Model file for the job. Use its own axes, mm. Coordinates: 2 decimals unless noted, no trailing zeros. Write each loop counter-clockwise with the first axis right and the second up, starting at its lowest first coordinate (ties: lowest second). Pieces come first, ordered by that corner, then holes. Notation, with made-up numbers: M 60,-20.5 L 72,-20.5 A24 ccw 72,9.5 Z; hole C 51,1.25 d10. An arc over 180 degrees is marked long. One line per question, with ' | ' between items. Start each with the question number.
(1) Cut at A-A (x = -267). Write the cut outline in (y, z).
(2) Flat gauge pins, fed straight in: pin 1 Ø0.8 at (x, y) = (-261.5, 1) entering from -Z; pin 2 Ø0.5 at (x, y) = (-262.5, 1) entering from +Z. Where does each tip first touch, or does it go through?
(3) Cut at C-C (z = -274). Write the cut outline in (x, y).
(4) Cut at B-B (x = -166.5). Write the cut outline in (y, z), plus the area to 3 significant figures.
(5) Wall check: probe 1 along X at (y, z) = (0.25, -95); probe 2 along Z at (x, y) = (-141.5, 0.9); probe 3 along Z at (x, y) = (-266, 0.4). Give the ranges that are in metal, low to high.
(6) Cut at D-D (y = 0.9). Count the separate pieces of the cut face and the enclosed holes in it, plus the area to 3 significant figures.
Autodesk Inventor part; units mm, degrees
ref_plane "YZ Plane" through (0, 0, 0) normal (1, 0, 0) x (0, 1, 0)
ref_plane "XZ Plane" through (0, 0, 0) normal (0, 1, 0) x (-1, 0, 0)
ref_plane "XY Plane" through (0, 0, 0) normal (0, 0, 1) x (1, 0, 0)
sketch "Sketch1" plane through (0, 0, 0) normal (0, 1, 0) x (-1, 0, 0)
  line L0 (0, 0) -> (355.6, 0)
  line L1 (355.6, 0) -> (355.6, -289.56)
  line L2 (355.6, -289.56) -> (0, -289.56)
  line L3 (0, -289.56) -> (0, 0)
  circle A0 centre (355.6, 0) radius 2.1082
  line L4 (355.6, 0) -> (361.95, 0)
  line L5 (355.6, 0) -> (355.6, 6.35)
  line L6 (355.6, 6.35) -> (361.95, 6.35)
  line L7 (0, -289.56) -> (0, -295.91)
  line L8 (0, -295.91) -> (-6.35, -295.91)
  line L9 (-6.35, -295.91) -> (361.95, -295.91)
  line L10 (361.95, -295.91) -> (361.95, 6.35)
  line L11 (361.95, 6.35) -> (-6.35, 6.35)
  line L12 (-6.35, 6.35) -> (-6.35, -295.91)
  circle A1 centre (355.6, -289.56) radius 2.1082
  circle A2 centre (0, -289.56) radius 2.1082
  circle A3 centre (0, 0) radius 2.1082
  line L13 (0, 0) -> (0, -20.32)
  line L14 (0, -20.32) -> (10.16, -20.32)
  line L15 (0, 0) -> (5.08, 0)
  line L16 (0, -289.56) -> (5.08, -289.56)
  line L17 (0, -289.56) -> (0, -269.24)
  line L18 (0, -269.24) -> (11.0826, -269.24)
  line L19 (355.6, 0) -> (355.6, -20.32)
  line L20 (355.6, -20.32) -> (345.44, -20.32)
  line L21 (355.6, 0) -> (350.52, 0)
  line L22 (355.6, -289.56) -> (350.52, -289.56)
  line L23 (355.6, -289.56) -> (355.6, -269.24)
  line L24 (355.6, -269.24) -> (345.44, -269.24)
  line L25 (345.44, -20.32) -> (10.16, -20.32)
  line L26 (355.6, -20.32) -> (355.6, -33.02)
  line L27 (355.6, -33.02) -> (0, -33.02)
  line L28 (355.6, -269.24) -> (355.6, -256.54)
  line L29 (355.6, -256.54) -> (0, -256.54)
  line L30 (345.44, -269.24) -> (11.0826, -269.24)
  line L31 (0, 0) -> (6.35, 0)
  arc A4 (6.35, 0) -> (10.16, -20.32) centre (82.4575, 3.753) ccw
  line L32 (6.35, 0) -> (-6.35, 0)
  line L33 (-6.35, 0) -> (-6.35, -289.56)
  line L34 (-6.35, -289.56) -> (6.35, -289.56)
  line L35 (6.35, -289.56) -> (6.35, 0)
  arc A5 (11.0826, -269.24) -> (6.35, -289.56) centre (82.2313, -296.5221) ccw
  line L36 (355.6, 0) -> (349.25, 0)
  line L37 (349.25, 0) -> (349.25, -289.56)
  arc A6 (349.25, -289.56) -> (345.44, -269.24) centre (298.4597, -288.566) ccw
  arc A7 (345.44, -20.32) -> (349.25, 0) centre (298.4597, -0.994) ccw
  line L38 (349.25, 0) -> (349.25, 6.35)
  line L39 (349.25, -289.56) -> (349.25, -295.91)
  line L40 (6.35, -289.56) -> (6.35, -295.91)
  line L41 (6.35, 0) -> (6.35, 6.35)
  dimension "d0" = 355.6
  dimension "d1" = 289.56
  dimension "d2" = 4.2164
  dimension "d3" = 6.35
  dimension "d4" = 6.35
  dimension "d5" = 6.35
  dimension "d6" = 6.35
  dimension "d7" = 20.32
  dimension "d8" = 10.16
  dimension "d10" = 20.32
  dimension "d12" = 20.32
  dimension "d13" = 10.16
  dimension "d16" = 5.08
  dimension "d17" = 20.32
  dimension "d18" = 10.16
  dimension "d20" = 12.7
  dimension "d21" = 12.7
  dimension "d23" = 6.35
  dimension "d24" = 76.2
  dimension "d25" = 76.2
  dimension "d26" = 6.35
  dimension "d27" = 50.8
  dimension "d28" = 50.8
extrude "Extrusion1" add sketch "Sketch1" along normal blind 1.5875 contours A3 L32 L12 L11 L41 L0 | L0 L35 L14 L3 A3 | L3 A2 L34 L12 L32 A3 | L14 L35 L27 L3 | A4 L14 L35 | L27 L35 L29 L3 | L14 L25 L20 L37 L27 L35 | L34 A2 L7 L8 L12 | L38 L11 L5 A0 L0 | L0 A0 L1 L20 L37 A7 | L29 L35 L18 L3 | L27 L37 L29 L35 | L37 L20 A7 | L18 L35 L2 A2 L3 | L29 L37 L24 L30 L18 L35 | L37 L20 L1 L27 | L27 L1 L29 L37 | L7 A2 L2 L40 L9 | L6 L10 L4 A0 L5 | L18 A5 L35 | L29 L1 L24 L37 | L1 A0 L4 L10 L9 L39 L2 A1 | L37 A6 L24 | L24 L1 A1 L2 A6 L37
sketch "Sketch2" plane through (0, 1.5875, 0) normal (0, 1, 0) x (1, 0, 0)
  circle A0 centre (-355.6, 289.56) radius 2.1082
  line L0 (-355.6, 289.56) -> (-355.6, 246.38)
  line L1 (-355.6, 246.38) -> (-284.48, 246.38)
  line L2 (-355.6, 289.56) -> (-355.6, 185.42)
  line L3 (-355.6, 185.42) -> (-223.52, 185.42)
  line L4 (-284.48, 246.38) -> (-223.52, 246.38)
  line L5 (-223.52, 246.38) -> (-223.52, 185.42)
  line L6 (-223.52, 185.42) -> (-284.48, 185.42)
  line L7 (-284.48, 185.42) -> (-284.48, 246.38)
  line L8 (-355.6, 289.56) -> (-355.6, 243.84)
  line L9 (-355.6, 243.84) -> (-220.98, 243.84)
  line L10 (-355.6, 289.56) -> (-355.6, 184.15)
  line L11 (-355.6, 289.56) -> (-355.6, 182.88)
  line L12 (-355.6, 182.88) -> (-160.02, 182.88)
  line L13 (-220.98, 243.84) -> (-160.02, 243.84)
  line L14 (-160.02, 243.84) -> (-160.02, 182.88)
  line L15 (-160.02, 182.88) -> (-220.98, 182.88)
  line L16 (-220.98, 182.88) -> (-220.98, 243.84)
  line L17 (-355.6, 289.56) -> (-355.6, 220.98)
  line L18 (-355.6, 220.98) -> (-157.48, 220.98)
  line L19 (-355.6, 289.56) -> (-355.6, 160.02)
  line L20 (-355.6, 160.02) -> (-96.52, 160.02)
  line L21 (-157.48, 220.98) -> (-96.52, 220.98)
  line L22 (-96.52, 220.98) -> (-96.52, 160.02)
  line L23 (-96.52, 160.02) -> (-157.48, 160.02)
  line L24 (-157.48, 160.02) -> (-157.48, 220.98)
  line L25 (-355.6, 289.56) -> (-81.28, 289.56)
  line L26 (-81.28, 289.56) -> (-81.28, 220.98)
  line L27 (-355.6, 289.56) -> (-20.32, 289.56)
  line L28 (-20.32, 289.56) -> (-20.32, 160.02)
  line L29 (-81.28, 220.98) -> (-20.32, 220.98)
  line L30 (-20.32, 220.98) -> (-20.32, 160.02)
  line L31 (-20.32, 160.02) -> (-81.28, 160.02)
  line L32 (-81.28, 160.02) -> (-81.28, 220.98)
  line L33 (-355.6, 289.56) -> (-160.02, 289.56)
  line L34 (-160.02, 289.56) -> (-160.02, 269.24)
  line L35 (-11.0826, 269.24) -> (-345.44, 269.24)
  line L36 (-160.02, 269.24) -> (-160.02, 256.54)
  line L37 (-160.02, 256.54) -> (6.35, 255.27)
  line L38 (6.35, -6.35) -> (6.35, 295.91)
  line L39 (6.35, 255.27) -> (-6.3496, 255.3669)
  line L40 (-160.02, 289.56) -> (-160.02, 231.14)
  line L41 (-6.3496, 255.3669) -> (-6.3496, 231.14)
  line L42 (-6.3496, 231.14) -> (-160.02, 231.14)
  line L43 (-160.02, 256.54) -> (-147.32, 256.54)
  line L44 (-147.32, 256.54) -> (-147.32, 231.14)
  line L45 (-147.32, 231.14) -> (-160.02, 231.14)
  line L46 (-160.02, 231.14) -> (-160.02, 256.54)
  line L47 (6.35, 295.91) -> (6.35, -6.35)
  line L48 (-361.95, 295.91) -> (-361.95, -6.35)
  line L49 (6.35, 144.78) -> (-361.95, 144.78)
  circle A1 centre (-355.6, 0) radius 2.1082
  line L50 (-355.6, 0) -> (-355.6, 43.18)
  line L51 (-355.6, 43.18) -> (-284.48, 43.18)
  line L52 (-355.6, 0) -> (-355.6, 104.14)
  line L53 (-355.6, 104.14) -> (-223.52, 104.14)
  line L54 (-284.48, 43.18) -> (-223.52, 43.18)
  line L55 (-223.52, 43.18) -> (-223.52, 104.14)
  line L56 (-223.52, 104.14) -> (-284.48, 104.14)
  line L57 (-284.48, 104.14) -> (-284.48, 43.18)
  line L58 (-355.6, 0) -> (-355.6, 45.72)
  line L59 (-355.6, 45.72) -> (-220.98, 45.72)
  line L60 (-355.6, 0) -> (-355.6, 105.41)
  line L61 (-355.6, 0) -> (-355.6, 106.68)
  line L62 (-355.6, 106.68) -> (-160.02, 106.68)
  line L63 (-220.98, 45.72) -> (-160.02, 45.72)
  line L64 (-160.02, 45.72) -> (-160.02, 106.68)
  line L65 (-160.02, 106.68) -> (-220.98, 106.68)
  line L66 (-220.98, 106.68) -> (-220.98, 45.72)
  line L67 (-355.6, 0) -> (-355.6, 68.58)
  line L68 (-355.6, 68.58) -> (-157.48, 68.58)
  line L69 (-355.6, 0) -> (-355.6, 129.54)
  line L70 (-355.6, 129.54) -> (-96.52, 129.54)
  line L71 (-157.48, 68.58) -> (-96.52, 68.58)
  line L72 (-96.52, 68.58) -> (-96.52, 129.54)
  line L73 (-96.52, 129.54) -> (-157.48, 129.54)
  line L74 (-157.48, 129.54) -> (-157.48, 68.58)
  line L75 (-355.6, 0) -> (-81.28, 0)
  line L76 (-81.28, 0) -> (-81.28, 68.58)
  line L77 (-355.6, 0) -> (-20.32, 0)
  line L78 (-20.32, 0) -> (-20.32, 129.54)
  line L79 (-81.28, 68.58) -> (-20.32, 68.58)
  line L80 (-20.32, 68.58) -> (-20.32, 129.54)
  line L81 (-20.32, 129.54) -> (-81.28, 129.54)
  line L82 (-81.28, 129.54) -> (-81.28, 68.58)
  line L83 (-355.6, 0) -> (-160.02, 0)
  line L84 (-160.02, 0) -> (-160.02, 20.32)
  line L85 (-11.0826, 20.32) -> (-345.44, 20.32)
  line L86 (-160.02, 20.32) -> (-160.02, 33.02)
  line L87 (-160.02, 33.02) -> (6.35, 34.29)
  line L88 (6.35, 34.29) -> (-6.3496, 34.1931)
  line L89 (-160.02, 0) -> (-160.02, 58.42)
  line L90 (-6.3496, 34.1931) -> (-6.3496, 58.42)
  line L91 (-6.3496, 58.42) -> (-160.02, 58.42)
  line L92 (-160.02, 33.02) -> (-147.32, 33.02)
  line L93 (-147.32, 33.02) -> (-147.32, 58.42)
  line L94 (-147.32, 58.42) -> (-160.02, 58.42)
  line L95 (-160.02, 58.42) -> (-160.02, 33.02)
  line L96 (-361.95, -6.35) -> (-361.95, 295.91)
  line L97 (-96.52, 160.02) -> (-81.28, 160.02)
  line L98 (-88.9, 160.02) -> (-88.9, 144.78)
  line L99 (-88.9, 144.78) -> (-88.9, 182.88)
  circle A2 centre (-88.9, 182.88) radius 1.778
  line L100 (-88.9, 144.78) -> (-88.9, 106.68)
  circle A3 centre (-88.9, 106.68) radius 1.778
  point P0 (0, 0)
  point P1 (-223.52, 243.84)
  point P2 (-284.48, 243.84)
  point P3 (-147.32, 256.4431)
  point P4 (-147.32, 33.1169)
  dimension "d31" = 43.18
  dimension "d32" = 71.12
  dimension "d33" = 104.14
  dimension "d34" = 132.08
  dimension "d35" = 45.72
  dimension "d36" = 134.62
  dimension "d37" = 105.41
  dimension "d38" = 106.68
  dimension "d39" = 195.58
  dimension "d42" = 68.58
  dimension "d43" = 198.12
  dimension "d44" = 129.54
  dimension "d45" = 259.08
  dimension "d46" = 274.32
  dimension "d47" = 68.58
  dimension "d49" = 335.28
  dimension "d50" = 129.54
  dimension "d51" = 195.58
  dimension "d52" = 12.7
  dimension "d53" = 12.7
  dimension "d54" = 58.42
  dimension "d55" = 12.7
  dimension "d56" = 38.1
  dimension "d57" = 3.556
  dimension "d58" = 38.1
  dimension "d59" = 3.556
extrude "Extrusion2" cut sketch "Sketch2" against normal blind 25.4 contours L87 L78 L91 L90 | A3 | L4 L5 L9 L7 | L9 L5 L18 L7 | L37 L28 L42 L26 | L26 L42 L44 L37 | L14 L18 L16 L13 | L18 L5 L3 L7 | A2 | L37 L41 L42 L28 | L29 L28 L31 L32 | L18 L14 L12 L16 | L21 L22 L20 L24 | L87 L76 L91 L78 | L87 L93 L91 L76 | L79 L82 L81 L78 | L64 L63 L66 L68 | L68 L66 L62 L64 | L74 L70 L72 L71 | L59 L57 L68 L55 | L55 L54 L57 L59 | L68 L57 L53 L55
properties part number "belly pan"
Filled in:
1) outline: M 0,-269.24 L 1.59,-269.24 L 1.59,-246.38 L 0,-246.38 Z; M 0,-185.42 L 1.59,-185.42 L 1.59,-104.14 L 0,-104.14 Z; M 0,-43.18 L 1.59,-43.18 L 1.59,-20.32 L 0,-20.32 Z
2) pin 1: z = -269.24 | pin 2: z = -20.32
3) outline: M -361.95,0 L -347.13,0 L -347.13,1.59 L -361.95,1.59 Z; M -9.44,0 L 6.35,0 L 6.35,1.59 L -9.44,1.59 Z
4) outline: M 0,-269.24 L 1.59,-269.24 L 1.59,-243.84 L 0,-243.84 Z; M 0,-182.88 L 1.59,-182.88 L 1.59,-106.68 L 0,-106.68 Z; M 0,-45.72 L 1.59,-45.72 L 1.59,-20.32 L 0,-20.32 Z | area: 202 mm²
5) probe 1: -361.95 to -284.48, -223.52 to -220.98, -160.02 to -157.48, -96.52 to -81.28, -20.32 to 6.35 | probe 2: -269.24 to -256.4, -231.14 to -220.98, -160.02 to -129.54, -68.58 to -58.42, -33.16 to -20.32 | probe 3: -269.24 to -246.38, -185.42 to -104.14, -43.18 to -20.32
6) separate pieces: 1 | enclosed holes: 16 | area: 56,400 mm²
